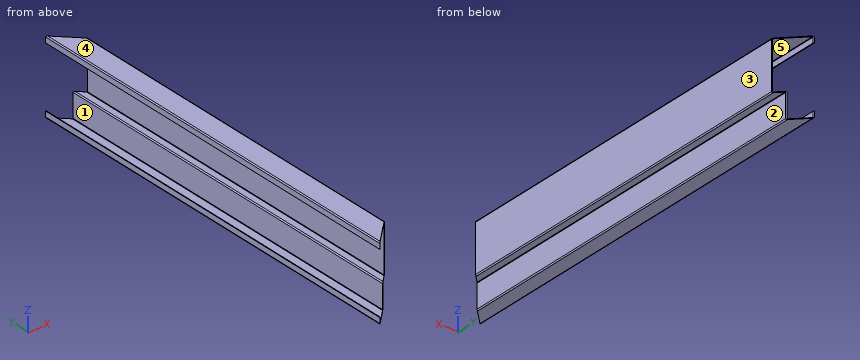
```python
from build123d import *

# Parameters (mm, degrees)
BASE_FLANGE1_DEPTH = 390.5
CUT_EXTRUDE2_DEPTH = 419.369827425


# Sheet-metal steps are written as plain solids
with BuildPart() as part:
    # Sketch1 → Base-Flange1 (new, symmetric)
    with BuildSketch(Plane(origin=(0, 0, 0), x_dir=(1, 0, 0), z_dir=(0, 1, 0))):
        with BuildLine():
            Line((9.5, 58), (9.5, 68.0134))
            ThreePointArc((9.5, 68.0134), (10.081861668, 69.418138332), (11.4866, 70))
            Line((11.4866, 70), (37.5134, 70))
            ThreePointArc((37.5134, 70), (38.918138332, 69.418138332), (39.5, 68.0134))
            Line((39.5, 68.0134), (39.5, 23.7366))
            ThreePointArc((39.5, 23.7366), (39.715745145, 23.215745145), (40.2366, 23))
            Line((40.2366, 23), (52.2634, 23))
            ThreePointArc((52.2634, 23), (53.668138332, 22.418138332), (54.25, 21.0134))
            Line((54.25, 21.0134), (54.25, 18))
            Line((54.25, 18), (54.25, -23))
            Line((54.25, -23), (54.25, -68.0134))
            ThreePointArc((54.25, -68.0134), (53.668138332, -69.418138332), (52.2634, -70))
            Line((52.2634, -70), (39.5, -70))
            Line((39.5, -70), (11.4866, -70))
            ThreePointArc((11.4866, -70), (10.081861668, -69.418138332), (9.5, -68.0134))
            Line((9.5, -68.0134), (9.5, -58))
            Line((9.5, -58), (10.75, -58))
            Line((10.75, -58), (10.75, -68.0134))
            ThreePointArc((10.75, -68.0134), (10.965745145, -68.534254855), (11.4866, -68.75))
            Line((11.4866, -68.75), (39.5, -68.75))
            Line((39.5, -68.75), (52.2634, -68.75))
            ThreePointArc((52.2634, -68.75), (52.784254855, -68.534254855), (53, -68.0134))
            Line((53, -68.0134), (53, -23))
            Line((53, -23), (53, 18))
            Line((53, 18), (53, 21.0134))
            ThreePointArc((53, 21.0134), (52.784254855, 21.534254855), (52.2634, 21.75))
            Line((52.2634, 21.75), (40.2366, 21.75))
            ThreePointArc((40.2366, 21.75), (38.831861668, 22.331861668), (38.25, 23.7366))
            Line((38.25, 23.7366), (38.25, 68.0134))
            ThreePointArc((38.25, 68.0134), (38.034254855, 68.534254855), (37.5134, 68.75))
            Line((37.5134, 68.75), (11.4866, 68.75))
            ThreePointArc((11.4866, 68.75), (10.965745145, 68.534254855), (10.75, 68.0134))
            Line((10.75, 68.0134), (10.75, 58))
            Line((10.75, 58), (9.5, 58))
        make_face()
    extrude(amount=BASE_FLANGE1_DEPTH, both=True)

    # Sketch2 → Cut-Extrude2 (cut, through all)
    with BuildSketch(Plane.XY.offset(70)):
        Polygon((9.5, -390.5), (204.29871247, -195.70128753), (123.087268974, -390.5), align=None)
        Polygon((123.087268974, 390.5), (9.5, 390.5), (204.29871247, 195.70128753), align=None)
    extrude(amount=-CUT_EXTRUDE2_DEPTH, mode=Mode.SUBTRACT)


solid = part.part
```
The model under review builds one solid part; all positions refer to its coordinate system, in mm. Face numbers are marked on the shaded views. A direction names the side the tool comes from. Give positions to 0.01 mm unless a question says otherwise; leave off trailing zeros. Write each loop counter-clockwise with the first axis right and the second up, starting at its lowest first coordinate (ties: lowest second). Pieces come first, ordered by that corner, then holes. Notation, with made-up numbers: (24.25, 35) -> (62.25, 35) arc R29 ccw to (62.25, 71) -> close; hole circle Ø3 at (-11.5, 79.25). An arc over 180 degrees is marked (long way). Answer in a Markdown table with one row per item.
1) For L1, parallel to Z at x = 35, y = 318.5; L2, parallel to X at y = 300.5, z = -62.5; L3, parallel to Z at x = 44, y = -176, list the stretches that pass through material, from the lowest coordinate up. Write a range as [from, to].
Worked answers:
| item | result |
|---|---|
| L1 | [-70, -68.75], [68.75, 70] |
| L2 | [9.5, 10.75], [38.25, 39.5] |
| L3 | [-23, -21.75], [68.75, 70] |
2) Clearance check with flat-ended pins moving along their axes: P1, Ø8, axis at y = 179.5, z = -62, coming from the +X side; P2, Ø1, axis at x = 41, y = 232, coming from the -Z side; P3, Ø1, axis at y = 273, z = 24.5, coming from the -X side. State where each tip first meets the part, or that it passes through.
Worked answers:
| item | result |
|---|---|
| P1 | x = 39.5 |
| P2 | z = -23 |
| P3 | x = 53 |
3) Add section C-C on z = -41.5. State the section outline as (x, y) points, plus the area to 3 significant figures.
Worked answers:
| item | result |
|---|---|
| outline | (38.25, -361.75) -> (39.5, -360.5) -> (39.5, 360.5) -> (38.25, 361.75) -> close |
| area | 903 mm² |
4) Add section B-B on y = -54. State the section outline as (x, z) points.
Worked answers:
| item | result |
|---|---|
| outline | (9.5, -68.01) arc R1.99 ccw to (11.49, -70) -> (37.51, -70) arc R1.99 ccw to (39.5, -68.01) -> (39.5, -23.74) arc R0.74 cw to (40.24, -23) -> (52.26, -23) arc R1.99 ccw to (54.25, -21.01) -> (54.25, 68.01) arc R1.99 ccw to (52.26, 70) -> (11.49, 70) arc R1.99 ccw to (9.5, 68.01) -> (9.5, 58) -> (10.75, 58) -> (10.75, 68.01) arc R0.74 cw to (11.49, 68.75) -> (52.26, 68.75) arc R0.74 cw to (53, 68.01) -> (53, -21.01) arc R0.74 cw to (52.26, -21.75) -> (40.24, -21.75) arc R1.99 ccw to (38.25, -23.74) -> (38.25, -68.01) arc R0.74 cw to (37.51, -68.75) -> (11.49, -68.75) arc R0.74 cw to (10.75, -68.01) -> (10.75, -58) -> (9.5, -58) -> close |
5) Tool access review of the marked faces 1 and 2: name each direction out of +Z, -Z, +X, -X, +Y, -Y from which nothing blocks a thin tool from reaching the whole face with its end or side.
Worked answers:
| item | result |
|---|---|
| face 1 | +Y, -Y |
| face 2 | -Z, +X, +Y, -Y |
6) Add section D-D on z = -13.5. State the section outline as (x, y) points.
Worked answers:
| item | result |
|---|---|
| outline | (53, -347) -> (54.25, -345.75) -> (54.25, 345.75) -> (53, 347) -> close |
7) Add section A-A on x = 29. State the section outline as (y, z) points, plus the area to 4 significant figures.
Worked answers:
| item | result |
|---|---|
| outline | (-371, -70) -> (371, -70) -> (371, -68.75) -> (-371, -68.75) -> close; (-371, 68.75) -> (371, 68.75) -> (371, 70) -> (-371, 70) -> close |
| area | 1,855 mm² |
8) Mouldability with a two-part tool opening along Z and no side actions: class the marked faces 3, 4 and 5 as +Z half, -Z half, draft (parallel to the pull), parting line (faces both ways), or undercut.
Worked answers:
| item | result |
|---|---|
| face 3 | draft |
| face 4 | +Z half |
| face 5 | undercut |
